Could you check a few things on this model? Use its own coordinates, in mm. A direction names the side the tool comes from. Coordinates: 2 decimals unless noted, no trailing zeros. Order: outer loops, then holes, each group sorted by start corner. A loop starts at its lowest first (then second) coordinate and runs counter-clockwise, first axis right, second up. Notation, with made-up numbers: (48, 48.5) -> (59, 48.5) arc R10 ccw to (59, 62.5) -> close; hole circle Ø5 at (31.25, 57). An arc over 180 degrees is marked (long way). Put each result on its own line as item: value. Start each with the question number.
Q1. Please list where these lines run through material, in increasing order: line 1 along Z through (x, y) = (50.2, 103.5); line 2 along Y through (x, z) = (35.5, 19.45); line 3 along Y through (x, z) = (35.5, 20.6).
Q2. We'd pull the mould along X, two halves only. Please class faces 5 (the face through (26.5, 81, 19)), 6 (the face through (33.6, 104.2, 19.2)), 7 (the face through (57, 54.5, 19)): +X half, -X half, draft (parallel to the pull), parting line (faces both ways), or undercut.
Q3. If we section it at C-C (x = 49): Please give me the cut outline in (y, z), and give its area (3 significant figures).
Q4. If we section it at D-D (x = 78.5): Please give me the cut outline in (y, z), and give its area (3 significant figures).
Q5. If we section it at A-A (y = 74.5): Please give me the cut outline in (x, z).
Q6. Will these pins go through, and if not, where does the flat tip stop? pin 1 (1 mm diameter, centred on x = 46.5, y = 77.5, fed in from -Z); pin 2 (4 mm diameter, centred on y = 69, z = 13.5, fed in from +X); pin 3 (10 mm diameter, centred on y = 81.5, z = 10.5, fed in from +X).
Q7. If we section it at B-B (z = 19): Please give me the cut outline in (x, y), and give its area (3 significant figures).
Q8. For faces 1 (the face through (37, 67, 18)), 2 (the face through (37, 101, 20.5)), 3 (the face through (74, 103, 18)), 4 (the face through (57, 82, 18)), which set-ups out of +Z, -Z, +X, -X, +Y, -Y let a thin tool reach every point of the face, with its end or its side?
from build123d import *

# Parameters (mm, degrees)
F_61_START                              = 18
F_61_X_61_RADAR_PLATFORM_DEPTH          = 3
C1_START                                = 17.9
C1_FOUR_CLEARANCES_43_X_43_MM_PROFILE_R = 1.4
C1_FOUR_CLEARANCES_43_X_43_MM_DEPTH     = 5.2
C1_SCREW_HEAD_POCKETS_PROFILE_R         = 2.55
C1_SCREW_HEAD_POCKETS_DEPTH             = 2.6
SKETCH_3_W                              = 5.8
SKETCH_3_H                              = 61
EXTRUDE_2_DEPTH                         = 16
SKETCH_4_R                              = 1.3
CUT_EXTRUDE_4_DEPTH                     = 25
SKETCH_5_W                              = 16
SKETCH_5_H                              = 17.8
EXTRUDE_3_DEPTH                         = 19
SKETCH_6_W                              = 19
SKETCH_6_H                              = 17.8
EXTRUDE_4_DEPTH                         = 16
CUT_EXTRUDE_5_DEPTH                     = 25.9
FILLET_4_R                              = 7
SKETCH_8_W                              = 61.060792307
SKETCH_8_H                              = 7.060792307
CUT_EXTRUDE_6_DEPTH                     = 25.9
FILLET_5_R                              = 5


with BuildPart() as part:
    # 61 x 61 radar platform profile → 61 x 61 radar platform (new body)
    with BuildSketch(Plane.XY.offset(F_61_START)):
        with BuildLine():
            Line((31.5, 47.5), (82.5, 47.5))
            ThreePointArc((82.5, 47.5), (86.035533906, 48.964466094), (87.5, 52.5))
            Line((87.5, 52.5), (87.5, 103.5))
            ThreePointArc((87.5, 103.5), (86.035533906, 107.035533906), (82.5, 108.5))
            Line((82.5, 108.5), (31.5, 108.5))
            ThreePointArc((31.5, 108.5), (27.964466094, 107.035533906), (26.5, 103.5))
            Line((26.5, 103.5), (26.5, 52.5))
            ThreePointArc((26.5, 52.5), (27.964466094, 48.964466094), (31.5, 47.5))
        make_face()
    extrude(amount=F_61_X_61_RADAR_PLATFORM_DEPTH)

    # C1 four clearances 43 x 43 mm profile → C1 four clearances 43 x 43 mm (cut)
    with BuildSketch(Plane.XY.offset(C1_START)):
        with Locations((35.5, 59.5)):
            Circle(C1_FOUR_CLEARANCES_43_X_43_MM_PROFILE_R)
        with Locations((35.5, 102.5)):
            Circle(C1_FOUR_CLEARANCES_43_X_43_MM_PROFILE_R)
        with Locations((78.5, 59.5)):
            Circle(C1_FOUR_CLEARANCES_43_X_43_MM_PROFILE_R)
        with Locations((78.5, 102.5)):
            Circle(C1_FOUR_CLEARANCES_43_X_43_MM_PROFILE_R)
    extrude(amount=C1_FOUR_CLEARANCES_43_X_43_MM_DEPTH, mode=Mode.SUBTRACT)

    # C1 screw head pockets profile → C1 screw head pockets (cut)
    with BuildSketch(Plane.XY.offset(C1_START)):
        with Locations((35.5, 59.5)):
            Circle(C1_SCREW_HEAD_POCKETS_PROFILE_R)
        with Locations((35.5, 102.5)):
            Circle(C1_SCREW_HEAD_POCKETS_PROFILE_R)
        with Locations((78.5, 59.5)):
            Circle(C1_SCREW_HEAD_POCKETS_PROFILE_R)
        with Locations((78.5, 102.5)):
            Circle(C1_SCREW_HEAD_POCKETS_PROFILE_R)
    extrude(amount=C1_SCREW_HEAD_POCKETS_DEPTH, mode=Mode.SUBTRACT)

    # 草图3 → 凸台-拉伸2 (add)
    with BuildSketch(Plane(origin=(0, 0, 18), x_dir=(-1, 0, 0), z_dir=(0, 0, -1))):
        with Locations((-63.1, 78)):
            Rectangle(SKETCH_3_W, SKETCH_3_H)
        with Locations((-50.9, 78)):
            Rectangle(SKETCH_3_W, SKETCH_3_H)
    extrude(amount=EXTRUDE_2_DEPTH)

    # 草图4 → 切除-拉伸4 (cut)
    with BuildSketch(Plane(origin=(66, 0, 0), x_dir=(0, 0, -1), z_dir=(1, 0, 0))):
        with Locations(Location((-15.5, 103.5, 0), (0, 0, 90))):
            Circle(SKETCH_4_R)
        with Locations(Location((-15.5, 74.5, 0), (0, 0, 90))):
            Circle(SKETCH_4_R)
        with Locations(Location((-5.5, 103.5, 0), (0, 0, 90))):
            Circle(SKETCH_4_R)
        with Locations(Location((-5.5, 74.5, 0), (0, 0, 90))):
            Circle(SKETCH_4_R)
    extrude(amount=-CUT_EXTRUDE_4_DEPTH, mode=Mode.SUBTRACT)

    # 草图5 → 凸台-拉伸3 (add)
    with BuildSketch(Plane(origin=(66, 0, 0), x_dir=(0, 0, -1), z_dir=(1, 0, 0))):
        with Locations((-10, 88)):
            Rectangle(SKETCH_5_W, SKETCH_5_H)
    extrude(amount=EXTRUDE_3_DEPTH)

    # 草图6 → 凸台-拉伸4 (add)
    with BuildSketch(Plane(origin=(0, 0, 18), x_dir=(-1, 0, 0), z_dir=(0, 0, -1))):
        with Locations((-38.5, 88)):
            Rectangle(SKETCH_6_W, SKETCH_6_H)
    extrude(amount=EXTRUDE_4_DEPTH)

    # 草图7 → 切除-拉伸5 (cut)
    with BuildSketch(Plane(origin=(0, 96.9, 0), x_dir=(1, 0, 0), z_dir=(0, 1, 0))):
        Polygon((66, -2), (85, -2), (85, -18), align=None)
        Polygon((48, -2), (29, -2), (29, -18), align=None)
    extrude(amount=-CUT_EXTRUDE_5_DEPTH, mode=Mode.SUBTRACT)

    # 圆角4
    # the kernel refuses this fillet: 7 mm, written as the material it adds along each edge
    with BuildSketch(Plane(origin=(85, 79.1, 18), x_dir=(-0.7649111981170483, 0, -0.6441357457827827), z_dir=(0, 1, 0))) as fillet_4_piece_1_section:
        with BuildLine():
            CenterArc((FILLET_4_R * 0.364967793547, -FILLET_4_R), FILLET_4_R, 90, 40.100907546)
            Line((-FILLET_4_R * 0.279167952236, -FILLET_4_R * 0.235088801883), (0, 0))
            Line((0, 0), (FILLET_4_R * 0.364967793547, 0))
        make_face()
    fillet_4_piece_1 = extrude(amount=17.8, mode=Mode.PRIVATE)
    fillet_4_piece_1 = split(fillet_4_piece_1, bisect_by=Plane(origin=(87.5, 88, 17.657135978), z_dir=(-1, 0, 0)), keep=Keep.TOP, mode=Mode.PRIVATE)
    add(fillet_4_piece_1)
    with BuildSketch(Plane(origin=(29, 96.9, 18), x_dir=(-1, 0, 0), z_dir=(0, -1, 0))) as fillet_4_piece_2_section:
        with BuildLine():
            CenterArc((FILLET_4_R * 0.364967793547, FILLET_4_R), FILLET_4_R, 229.899092454, 40.100907546)
            Line((-FILLET_4_R * 0.279167952236, FILLET_4_R * 0.235088801883), (0, 0))
            Line((0, 0), (FILLET_4_R * 0.364967793547, 0))
        make_face()
    fillet_4_piece_2 = extrude(amount=17.8, mode=Mode.PRIVATE)
    fillet_4_piece_2 = split(fillet_4_piece_2, bisect_by=Plane(origin=(26.5, 88, 17.657135978), z_dir=(1, 0, 0)), keep=Keep.TOP, mode=Mode.PRIVATE)
    add(fillet_4_piece_2)

    # 草图8 → 切除-拉伸6 (cut)
    with BuildSketch(Plane.XY.offset(21)):
        with Locations((57.030396153, 50.969603847)):
            Rectangle(SKETCH_8_W, SKETCH_8_H)
    extrude(amount=-CUT_EXTRUDE_6_DEPTH, mode=Mode.SUBTRACT)

    # 圆角5
    fillet_5_edges = [part.edges().sort_by_distance(p)[0] for p in [
        (63.1, 54.5, 2),
        (26.5, 54.5, 19.5),
        (87.5, 54.5, 19.5),
        (50.9, 54.5, 2),
        (63.1, 108.5, 2),
        (50.9, 108.5, 2),
    ]]
    fillet(fillet_5_edges, radius=FILLET_5_R)


solid = part.part
The answers:
1. line 1: 2 to 4.2, 6.8 to 14.2, 16.8 to 21
1. line 2: 54.5 to 56.95, 62.05 to 99.95, 105.05 to 108.5
1. line 3: 54.5 to 58.1, 60.9 to 101.1, 103.9 to 108.5
2. face 5: -X half
2. face 6: undercut
2. face 7: draft
3. outline: (54.5, 7) arc R5 ccw to (59.5, 2) -> (103.5, 2) arc R5 ccw to (108.5, 7) -> (108.5, 21) -> (54.5, 21) -> close; hole circle Ø2.6 at (74.5, 5.5); hole circle Ø2.6 at (74.5, 15.5); hole circle Ø2.6 at (103.5, 5.5); hole circle Ø2.6 at (103.5, 15.5)
3. area: 994 mm^2
4. outline: (54.5, 18) -> (56.95, 18) -> (56.95, 20.5) -> (58.1, 20.5) -> (58.1, 21) -> (54.5, 21) -> close; (60.9, 20.5) -> (62.05, 20.5) -> (62.05, 18) -> (79.1, 18) -> (79.1, 12.53) -> (96.9, 12.53) -> (96.9, 18) -> (99.95, 18) -> (99.95, 20.5) -> (101.1, 20.5) -> (101.1, 21) -> (60.9, 21) -> close; (103.9, 20.5) -> (105.05, 20.5) -> (105.05, 18) -> (108.5, 18) -> (108.5, 21) -> (103.9, 21) -> close
4. area: 231 mm^2
5. outline: (26.5, 18) -> (48, 18) -> (48, 16.8) -> (53.8, 16.8) -> (53.8, 18) -> (60.2, 18) -> (60.2, 16.8) -> (66, 16.8) -> (66, 18) -> (87.5, 18) -> (87.5, 21) -> (26.5, 21) -> close; (48, 2) -> (53.8, 2) -> (53.8, 4.2) -> (48, 4.2) -> close; (48, 6.8) -> (53.8, 6.8) -> (53.8, 14.2) -> (48, 14.2) -> close; (60.2, 2) -> (66, 2) -> (66, 4.2) -> (60.2, 4.2) -> close; (60.2, 6.8) -> (66, 6.8) -> (66, 14.2) -> (60.2, 14.2) -> close
6. pin 1: z = 18
6. pin 2: x = 66
6. pin 3: x = 82.03
7. outline: (26.5, 59.5) arc R5 ccw to (31.5, 54.5) -> (82.5, 54.5) arc R5 ccw to (87.5, 59.5) -> (87.5, 103.5) arc R5 ccw to (82.5, 108.5) -> (31.5, 108.5) arc R5 ccw to (26.5, 103.5) -> close; hole circle Ø5.1 at (35.5, 59.5); hole circle Ø5.1 at (35.5, 102.5); hole circle Ø5.1 at (78.5, 59.5); hole circle Ø5.1 at (78.5, 102.5)
7. area: 3,190 mm^2
8. face 1: -Z, -X, -Y
8. face 2: -Z
8. face 3: -Z, +X, +Y
8. face 4: -Z, +Y, -Y
